Design review of the part built by this model. Coordinates are the model's own, in mm. A direction names the side the tool comes from. Coordinates: 2 decimals unless noted, no trailing zeros. Loops run counter-clockwise (first coordinate to the right, second up) from the corner with the lowest first, then second, coordinate; pieces in that order, holes last.
Q1. Wall thickness on probe 1 along Y at (x, z) = (-12.5, 10); probe 2 along Z at (x, y) = (29.6, 22.95); probe 3 along X at (y, z) = (5, 10.5): over which ranges is each line inside the solid? List them lowest first.
Q2. Add section D-D on z = 2.5. Give the boundary of the cut face in (x, y).
Q3. Add section B-B on y = 7.25. Give the boundary of the cut face in (x, z).
Q4. Machinability: for faces 4 (the face through (-15, 3, 4.25)), 5 (the face through (12.1, 23, 6)), 6 (the face through (-16.7, 19, 6)), which of the approach directions +Z, -Z, +X, -X, +Y, -Y give a long, thin tool a straight path to every point of the face, cutting with its end or side? Answer none if there is none.
Q5. Add section C-C on z = 6. Give the number of separate pieces and of enclosed holes in the cut face, and give its area (3 significant figures).
Q6. Add section A-A on x = -15.5. Give the boundary of the cut face in (y, z).
Q7. For P1, Ø3, axis at x = -29.6, z = 6, coming from the +Y side; P2, Ø6, axis at y = 9, z = 6, coming from the +X side; P3, Ø3.5, axis at x = -27, z = 4, coming from the -Y side; P4, Ø3.5, axis at y = 11.5, z = 5, coming from the -X side, all flat-tipped, find the tip position at first contact; note any pin that passes through.
Q8. Draft analysis for pull direction Y (two halves, no side actions). For faces 1 (the face through (-15, 3, 11)), 2 (the face through (14, 11, 12)), 3 (the face through (23, 25, 6)), state which applies: released by +Y, released by -Y, zero draft, split by the parting line, or undercut.
```python
from build123d import *

# Parameters (mm, degrees)
SALIENTE_EXTRUIR1_DEPTH = 12
CORTAR_EXTRUIR1_DEPTH   = 8
CROQUIS4_W              = 6.6
CROQUIS4_H              = 2.892350448
SALIENTE_EXTRUIR3_DEPTH = 3
CROQUIS2_W              = 22.5
CROQUIS2_H              = 12
CROQUIS2_R              = 1.75
SALIENTE_EXTRUIR4_DEPTH = 3


with BuildPart() as part:
    # Croquis1 → Saliente-Extruir1 (new body)
    with BuildSketch(Plane.XY):
        Polygon((-12.1, 0), (12.1, 0), (12.1, 17.5), (16.7, 17.5), (16.7, 20.5), (12.1, 20.5), (12.1, 25), (18.7, 25), (18.7, -2), (-18.7, -2), (-18.7, 25), (-12.1, 25), (-12.1, 20.5), (-16.7, 20.5), (-16.7, 17.5), (-12.1, 17.5), align=None)
    extrude(amount=SALIENTE_EXTRUIR1_DEPTH)

    # Croquis3 → Cortar-Extruir1 (cut)
    with BuildSketch(Plane(origin=(-12.1, 0, 0), x_dir=(0, 0, -1), z_dir=(1, 0, 0))):
        Polygon((-4.25, 0), (-7.75, 0), (-12, 0), (-12, 6), (-7.75, 6), (-4.25, 6), align=None)
    extrude(amount=-CORTAR_EXTRUIR1_DEPTH, mode=Mode.SUBTRACT)

    # Croquis4 → Saliente-Extruir3 (add)
    with BuildSketch(Plane.XZ.offset(-6)):
        with Locations((-15.4, 10.553824776)):
            Rectangle(CROQUIS4_W, CROQUIS4_H)
    extrude(amount=SALIENTE_EXTRUIR3_DEPTH)

    # Croquis2 → Saliente-Extruir4 (add)
    # profile 1 of 2: a face of its own
    with BuildSketch(Plane(origin=(0, 25, 0), x_dir=(1, 0, 0), z_dir=(0, 1, 0))):
        with Locations((-23.35, -6)):
            Rectangle(CROQUIS2_W, CROQUIS2_H)
        with Locations(Location((-29.6, -6, 0), (0, 0, 180))):
            Circle(CROQUIS2_R, mode=Mode.SUBTRACT)
    # profile 2 of 2: a face of its own
    with BuildSketch(Plane(origin=(0, 25, 0), x_dir=(1, 0, 0), z_dir=(0, 1, 0))):
        with Locations((23.35, -6)):
            Rectangle(CROQUIS2_W, CROQUIS2_H)
        with Locations(Location((29.6, -6, 0), (0, 0, 180))):
            Circle(CROQUIS2_R, mode=Mode.SUBTRACT)
    extrude(amount=-SALIENTE_EXTRUIR4_DEPTH)


solid = part.part
```
Entries:
1. probe 1: y = -2 to 0, 3 to 17.5, 20.5 to 25
1. probe 2: z = 0 to 4.25, 7.75 to 12
1. probe 3: x = -18.7 to -12.1, 12.1 to 18.7
2. outline: (-34.6, 22) - (-18.7, 22) - (-18.7, -2) - (18.7, -2) - (18.7, 22) - (34.6, 22) - (34.6, 25) - (12.1, 25) - (12.1, 20.5) - (16.7, 20.5) - (16.7, 17.5) - (12.1, 17.5) - (12.1, 0) - (-12.1, 0) - (-12.1, 17.5) - (-16.7, 17.5) - (-16.7, 20.5) - (-12.1, 20.5) - (-12.1, 25) - (-34.6, 25) - close
3. outline: (-18.7, 0) - (-12.1, 0) - (-12.1, 12) - (-18.7, 12) - close; (12.1, 0) - (18.7, 0) - (18.7, 12) - (12.1, 12) - close
4. face 4: -X
4. face 5: +Z, -Z, +Y
4. face 6: +Z, -Z
5. separate pieces: 4
5. enclosed holes: 0
5. area: 412 mm2
6. outline: (-2, 0) - (17.5, 0) - (17.5, 12) - (3, 12) - (3, 9.11) - (6, 9.11) - (6, 4.25) - (0, 4.25) - (0, 12) - (-2, 12) - close; (20.5, 0) - (25, 0) - (25, 12) - (20.5, 12) - close
7. P1: passes through
7. P2: stops at x = 18.7
7. P3: stops at y = 22
7. P4: stops at x = -18.7
8. face 1: undercut
8. face 2: zero draft
8. face 3: released by +Y
